Verification items for the finished model (mm, model axes). A direction names the side the tool comes from. Round coordinates to 2 decimals unless told otherwise and drop trailing zeros. Loops run counter-clockwise (first coordinate to the right, second up) from the corner with the lowest first, then second, coordinate; pieces in that order, holes last.
from build123d import *

# Parameters (mm, degrees)
SKETCH2_R           = 4
BOSS_EXTRUDE1_DEPTH = 3.175


with BuildPart() as part:
    # Sketch2 → Boss-Extrude1 (new body)
    with BuildSketch(Plane.XY):
        Polygon((-5, -11.5), (-1.5, -11.5), (-1.5, -8.325), (1.5, -8.325), (1.5, -11.5), (5, -11.5), (5, 11.5), (1.5, 11.5), (-1.5, 11.5), (-5, 11.5), (-5, 9.5), (-8.175, 9.5), (-8.175, -2.5), (-5, -2.5), align=None)
        with Locations((-1, 4.5)):
            Circle(SKETCH2_R, mode=Mode.SUBTRACT)
    extrude(amount=-BOSS_EXTRUDE1_DEPTH)


solid = part.part
1. Scan lines: L1, parallel to Y at x = -1, z = -1.3 (3 decimals); L2, parallel to Y at x = -7, z = -1.5; L3, parallel to Y at x = -2.5, z = -2.15. Record each from-to range of solid material in increasing order.
2. Tool access check on faces 4 (the face through (-2, 0, -3.175)), 5 (the face through (0, -8.325, -2)), 6 (the face through (-5, 11, -2)), 7 (the face through (-5, -7, -2)). Record the directions out of +Z, -Z, +X, -X, +Y, -Y that give a thin tool (end or side, any length) a straight path to the whole face; none if there is none.
3. Section check C-C (z = -0.4). Enter the section's corners in (x, y) (3 decimals), then the cut area to 3 significant figures.
4. Release check for a two-part mould opening along X. For faces 1 (the face through (3, -11.5, -2)), 2 (the face through (1.5, -10, -2)), 3 (the face through (5, 0, -2)) record: released by +X, released by -X, zero draft, split by the parting line, or undercut.
5. Gauge pin test, flat ends, axial feed: P1, Ø1.6, axis at x = -6.5, z = -2, coming from the +Y side; P2, Ø1.5, axis at y = -7, z = -2.5, coming from the -X side. Record the tip position at first contact, or that the pin passes through.
6. Section check D-D (x = -5.75). Enter the section's corners in (y, z) (3 decimals).
7. Section check B-B (y = 4.5). Enter the section's corners in (x, z) (3 decimals), then the cut area to 3 significant figures.
8. Section check A-A (x = -1). Enter the section's corners in (y, z) (3 decimals).
Taken from the geometry:
1. L1: y = -8.325 to 0.5, 8.5 to 11.5
1. L2: y = -2.5 to 9.5
1. L3: y = -11.5 to 0.79, 8.21 to 11.5
2. face 4: -Z, +X, -X, +Y, -Y
2. face 5: +Z, -Z, -Y
2. face 6: +Z, -Z, -X, +Y
2. face 7: +Z, -Z, -X, -Y
3. outline: (-8.175, -2.5) - (-5, -2.5) - (-5, -11.5) - (-1.5, -11.5) - (-1.5, -8.325) - (1.5, -8.325) - (1.5, -11.5) - (5, -11.5) - (5, 11.5) - (-5, 11.5) - (-5, 9.5) - (-8.175, 9.5) - close; hole circle Ø8 at (-1, 4.5)
3. area: 208 mm2
4. face 1: zero draft
4. face 2: undercut
4. face 3: released by +X
5. P1: stops at y = 9.5
5. P2: stops at x = -5
6. outline: (-2.5, -3.175) - (9.5, -3.175) - (9.5, 0) - (-2.5, 0) - close
7. outline: (-8.175, -3.175) - (-5, -3.175) - (-5, 0) - (-8.175, 0) - close; (3, -3.175) - (5, -3.175) - (5, 0) - (3, 0) - close
7. area: 16.4 mm2
8. outline: (-8.325, -3.175) - (0.5, -3.175) - (0.5, 0) - (-8.325, 0) - close; (8.5, -3.175) - (11.5, -3.175) - (11.5, 0) - (8.5, 0) - close
